Build history of the part. All positions in model axes, mm. A direction names the side the tool comes from. Coordinates: 2 decimals unless noted, no trailing zeros. Order: outer loops, then holes, each group sorted by start corner. A loop starts at its lowest first (then second) coordinate and runs counter-clockwise, first axis right, second up. Notation, with made-up numbers: M 24,62 L 56,62 A37 cw 56,98 Z; hole C 49.5,85 d3. An arc over 180 degrees is marked long. Use a Markdown table: item, result. Add a question column.
from build123d import *

# Parameters (mm, degrees)
F4_DEPTH     = 0.2
F5_COUNT     = 4
F8_DEPTH     = 6.0416666667
F9_T4_ANGLE  = 67.1804235359
F9_S7_R      = 0.25
F9_T8_DEPTH  = 2
F9_T12_ANGLE = 67.1804235359
F9_S15_R     = 0.25
F9_T16_DEPTH = 2


# Not quite as in the source:
# - a fillet or chamfer that OpenCascade refuses, or shapes differently, is made with other operations: its cross-section is extruded or revolved along the edge and cut away or added


with BuildPart() as f2:
    # F1 (on Front) → F2 (revolve)
    with BuildSketch(Plane.XZ):
        with BuildLine():
            Line((0, 25.6944444444), (0, 0))
            Line((0, 0), (0.7986111111, 0))
            Line((0.7986111111, 0), (0.7986111111, 23.4375))
            ThreePointArc((0.7986111111, 23.4375), (0.7106013269, 24.425281766), (0.4493446353, 25.3819444444))
            ThreePointArc((0.4493446353, 25.3819444444), (0.2736635029, 25.6086390085), (0, 25.6944444444))
        make_face()
    revolve(axis=Axis((0, 0, 12.8472222222), (0, 0, 1)))

    # F3 (on Front) → F4 (join, symmetric)
    with BuildSketch(Plane.XZ):
        Polygon((0, 23.8888888889), (0, 0), (0.7986111111, 0), (2.6736111111, 0), (2.6736111111, 3.125), (1.7361111111, 6.7013888889), (0.4, 7.9385288066), (0.4, 15.9410660661), (3.3680555556, 15.1388888889), (3.0208333333, 17.9166666667), (0.4, 17.343359375), (0.4, 19.7922705314), (1.5972222222, 20.8333333333), (1.5972222222, 22.6388888889), align=None)
    extrude(amount=F4_DEPTH, both=True)

    # F5: F2 ×4 about axis
    f5_axis = Axis((0, 0, 0), (0, 0, 1))


with BuildPart() as f2_1:
    add(f2.part)
    for i in range(1, F5_COUNT):
        add(f2.part.rotate(f5_axis, i * 360 / F5_COUNT))

    # F7 (on offset) → F8 (join)
    with BuildSketch(Plane.XY.offset(15.4166666667)):
        with BuildLine():
            Line((-0.4086259328, -0.7035839656), (-0.1424359704, -0.4373940032))
            Line((-0.1424359704, -0.4373940032), (-0.4373940032, -0.1424359704))
            Line((-0.4373940032, -0.1424359704), (-0.7035839656, -0.4086259328))
            ThreePointArc((-0.7035839656, -0.4086259328), (-0.6354140103, -0.6354140103), (-0.4086259328, -0.7035839656))
        make_face()
    extrude(amount=F8_DEPTH)

    # F9: chamfer of 0.1 on 2 edges, made by hand


with BuildPart() as f9_tool2:
    # F9_s3 → F9_t4 (revolve)
    with BuildSketch(Plane(origin=(0, 0, 0), x_dir=(0, 0, 1), z_dir=(-0.197824804, 0.9802373932, 0))):
        Polygon((21.5583333333, -0.7986111111), (21.4583333333, -0.8986111111), (21.4583333333, -0.7986111111), align=None)
    revolve(axis=Axis((0, 0, 21.4583333333), (0, 0, 1)), revolution_arc=F9_T4_ANGLE)

    split(bisect_by=Plane(origin=(0.1474790164, -0.1474790164, 0), x_dir=(0, 0, 1), z_dir=(-0.7071067812, 0.7071067812, 0)), keep=Keep.TOP)

    split(bisect_by=Plane(origin=(-0.1474790164, 0.1474790164, 0), x_dir=(0, 0, 1), z_dir=(0.7071067812, -0.7071067812, 0)), keep=Keep.TOP)

    # F9_s7 → F9_t8 (intersect, symmetric)
    with BuildSketch(Plane.XY.offset(21.5)):
        with Locations((-0.458637315, -0.458637315)):
            Circle(F9_S7_R)
    extrude(amount=F9_T8_DEPTH, both=True, mode=Mode.INTERSECT)


with BuildPart() as f2_2:
    add(f2_1.part)

    # F9_t1: union F9_tool2
    add(f9_tool2.part)


with BuildPart() as f9_tool10:
    # F9_s11 → F9_t12 (revolve)
    with BuildSketch(Plane(origin=(0, 0, 0), x_dir=(0, 0, 1), z_dir=(-0.197824804, 0.9802373932, 0))):
        Polygon((15.3166666667, -0.7986111111), (15.4166666667, -0.8986111111), (15.4166666667, -0.7986111111), align=None)
    revolve(axis=Axis((0, 0, 15.4166666667), (0, 0, 1)), revolution_arc=F9_T12_ANGLE)

    split(bisect_by=Plane(origin=(0.1474790164, -0.1474790164, 0), x_dir=(0, 0, 1), z_dir=(-0.7071067812, 0.7071067812, 0)), keep=Keep.TOP)

    split(bisect_by=Plane(origin=(-0.1474790164, 0.1474790164, 0), x_dir=(0, 0, 1), z_dir=(0.7071067812, -0.7071067812, 0)), keep=Keep.TOP)

    # F9_s15 → F9_t16 (intersect, symmetric)
    with BuildSketch(Plane.XY.offset(15.4)):
        with Locations((-0.458637315, -0.458637315)):
            Circle(F9_S15_R)
    extrude(amount=F9_T16_DEPTH, both=True, mode=Mode.INTERSECT)


with BuildPart() as f2_3:
    add(f2_2.part)

    # F9_t9: union F9_tool10
    add(f9_tool10.part)


solid = f2_3.part
(1) Slice it at A-A on x = -2. Give the cut face in (y, z), and give its area (3 significant figures).
(2) Drill centre lines: line 1 along Y through (x, z) = (-1, 1); line 2 along Z through (x, y) = (1.5, 0). Where is each one in solid material? Low to high. Write a range as from..to.
(3) Which spindle directions (+Z, -Z, +X, -X, +Y, -Y) get a long thin tool onto all of the face, cutting with end or side? Do faces 1 (the flat face through (-0.2, -1, 3)), 2 (the flat face through (-1, 0.2, 3)), 3 (the flat face through (2, 0.2, 17)), 4 (the flat face through (-2.21, 0, 4.89)). Say none if no direction does.
(4) Slice it at D-D on z = 3.5. Give the cut face in (x, y).
(5) Mould opens along Z. For faces 5 (the cylindrical face through (0.76, 0.24, 11.88)), 6 (the flat face through (-1, 0.2, 22)) say: released by +Z, released by -Z, zero draft, split by the parting line, or undercut.
(6) Drop flat-ended pins along their axis: P1, Ø4, axis at y = 2.5, z = 11, coming from the +X side; P2, Ø2, axis at y = -1.5, z = 3, coming from the -X side; P3, Ø3, axis at y = -2.5, z = 16, coming from the +X side. Give the stop position or say it passes through.
Solutions:
| question | item | result |
|---|---|---|
| 1 | outline | M -0.2,0 L 0.2,0 L 0.2,5.69 L -0.2,5.69 Z; M -0.2,15.51 L 0.2,15.51 L 0.2,17.69 L -0.2,17.69 Z |
| 1 | area | 3.15 mm² |
| 2 | line 1 | -0.2..0.2 |
| 2 | line 2 | 0..6.92, 15.64..17.58, 20.75..22.71 |
| 3 | face 1 | +Z, -Z, -X, -Y |
| 3 | face 2 | +Z, -Z, -X, +Y |
| 3 | face 3 | +Z, -Z, +X, +Y |
| 3 | face 4 | -X, +Y, -Y |
| 4 | outline | M -2.58,-0.2 L -0.77,-0.2 A0.8 ccw -0.2,-0.77 L -0.2,-2.58 L 0.2,-2.58 L 0.2,-0.77 A0.8 ccw 0.77,-0.2 L 2.58,-0.2 L 2.58,0.2 L 0.77,0.2 A0.8 ccw 0.2,0.77 L 0.2,2.58 L -0.2,2.58 L -0.2,0.77 A0.8 ccw -0.77,0.2 L -2.58,0.2 Z |
| 5 | face 5 | undercut |
| 5 | face 6 | zero draft |
| 6 | P1 | x = 0.62 |
| 6 | P2 | x = -0.62 |
| 6 | P3 | x = 0.2 |
